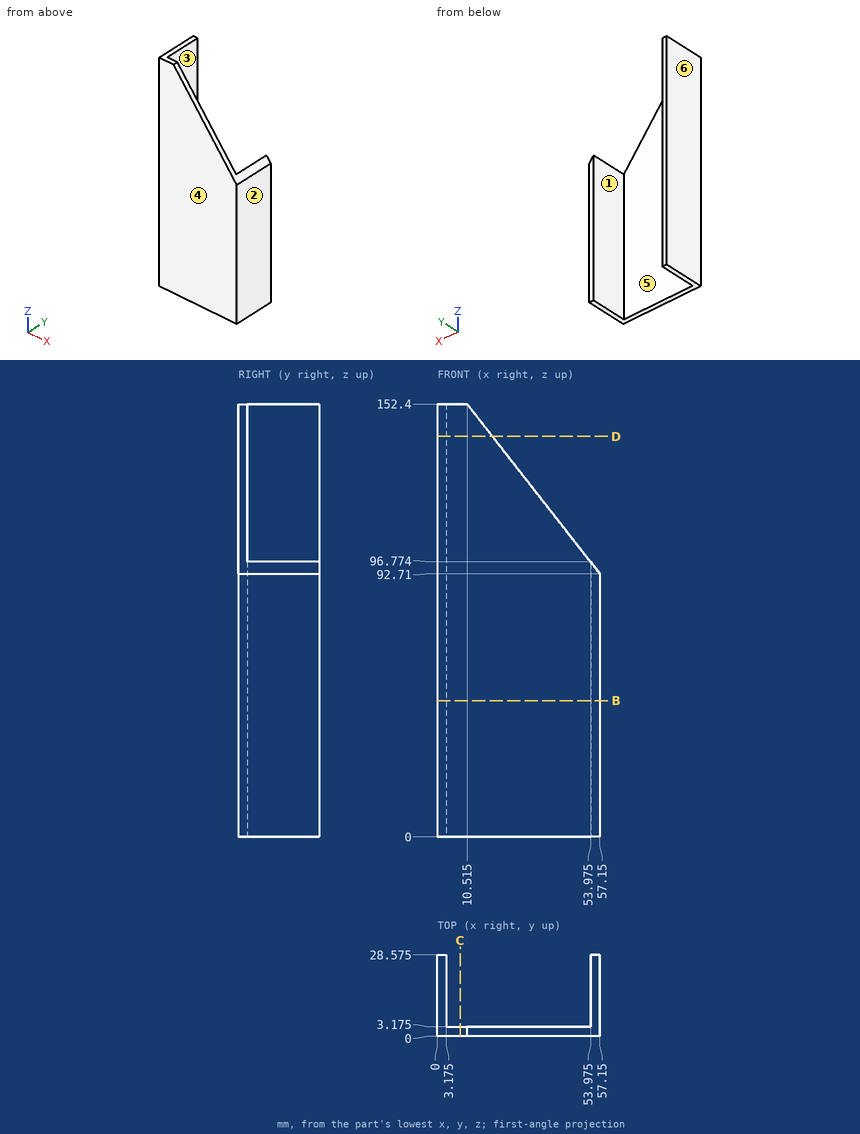
Here's the drawing with two shaded views (mm, measured from the low corner). I have some questions. A direction names the side the tool comes from. Give positions to 0.01 mm unless a question says otherwise; leave off trailing zeros. Write each loop counter-clockwise with the first axis right and the second up, starting at its lowest first coordinate (ties: lowest second). Pieces come first, ordered by that corner, then holes. Notation, with made-up numbers: (19, 66) -> (32, 66) arc R22 ccw to (32, 97) -> close; hole circle Ø9 at (-26, -21). An arc over 180 degrees is marked (long way). Answer as a JSON object with one key per item and string values. Group by question number.
Item 1: We'd pull the mould along X, two halves only. Please class the marked faces 3, 4, 5 and 6: +X half, -X half, draft (parallel to the pull), parting line (faces both ways), or undercut.
Item 2: Suppose I cut it at B-B (z = 48). Please give me the cut outline in (x, y) (3 decimals), plus the area to 3 significant figures.
Item 3: I'm going to push flat-ended pins straight in: P1, Ø5, axis at y = 15, z = 112.5, coming from the +X side (3 decimals); P2, Ø5, axis at x = 49, y = 19.5, coming from the +Z side; P3, Ø15, axis at x = 40.5, z = 86.5, coming from the +Y side (3 decimals). Where does each tip first touch, or does it pass through?
Item 4: Suppose I cut it at D-D (z = 141). Please give me the cut outline in (x, y) (1 decimal), plus the area to 3 significant figures.
Item 5: Suppose I cut it at C-C (x = 8). Please give me the cut outline in (y, z) (3 decimals).
Item 6: Please list where these lines run through material, in increasing order: line 1 (X direction, y = 26.75, z = 37.5) (3 decimals); line 2 (Y direction, x = 31, z = 126) (3 decimals). Write a range as [from, to].
Item 7: For the marked faces 1 and 2, which set-ups out of +Z, -Z, +X, -X, +Y, -Y let a thin tool reach every point of the face, with its end or its side?
Findings:
{
 "1": {"face 3": "undercut", "face 4": "draft", "face 5": "undercut", "face 6": "-X half"},
 "2": {"outline": "(0, 0) -> (57.15, 0) -> (57.15, 28.575) -> (53.975, 28.575) -> (53.975, 3.175) -> (3.175, 3.175) -> (3.175, 28.575) -> (0, 28.575) -> close", "area": "343 mm²"},
 "3": {"P1": "stops at x = 3.175", "P2": "passes through", "P3": "stops at y = 3.175"},
 "4": {"outline": "(0, 0) -> (19.4, 0) -> (19.4, 3.2) -> (3.2, 3.2) -> (3.2, 28.6) -> (0, 28.6) -> close", "area": "142 mm²"},
 "5": {"outline": "(0, 0) -> (3.175, 0) -> (3.175, 152.4) -> (0, 152.4) -> close"},
 "6": {"line 1": "x = [0, 3.175], [53.975, 57.15]", "line 2": "y = [0, 3.175]"},
 "7": {"face 1": "+Z, -Z, +Y", "face 2": "+Z, -Z, +X, +Y, -Y"}
}
